For this review, take the finished solid that the model builds, in its own axes (mm). A direction names the side the tool comes from. Round coordinates to 2 decimals unless told otherwise and drop trailing zeros. Write each loop counter-clockwise with the first axis right and the second up, starting at its lowest first coordinate (ties: lowest second). Pieces come first, ordered by that corner, then holes. Notation, with made-up numbers: (49.25, -5) -> (97.25, -5) arc R19 cw to (97.25, 11) -> close; hole circle Ø3 at (67.25, 37). An arc over 180 degrees is marked (long way). Answer as CSV lines item,"result". Start each with the question number.
Item 1: Take a section at D-D on z = -15. Give the boundary of the cut face in (x, y).
Item 2: Take a section at C-C on y = 20.5. Give the boundary of the cut face in (x, z), then the cut area to 3 significant figures.
Item 3: Machinability: for faces 4 (the flat face through (-12, 87, -36.799)), 5 (the flat face through (-10, 11.43, -28)), 6 (the flat face through (-12, 87, -17.749)), which of the approach directions +Z, -Z, +X, -X, +Y, -Y give a long, thin tool a straight path to every point of the face, cutting with its end or side? Answer none if there is none.
Item 4: Take a section at B-B on z = -23. Give the boundary of the cut face in (x, y), then the cut area to 3 significant figures.
Item 5: For pin 1 Ø8 at (y, z) = (43.5, -40.5) entering from +X; pin 2 Ø7 at (x, y) = (-12, 84.5) entering from -Z; pin 3 Ø10 at (x, y) = (-9, 85.5) entering from +Z, all flat-tipped, find the tip position at first contact; note any pin that passes through.
Item 6: Wall thickness on probe 1 along Y at (x, z) = (-16, -25); probe 2 along X at (y, z) = (70, -52); probe 3 along Y at (x, z) = (-16.5, -15): over which ranges is each line inside the solid? List them lowest first. Write a range as from..to.
Item 7: Mouldability with a two-part tool opening along Y and no side actions: class faces 1 (the flat face through (-5.08, 87, -27)), 2 (the flat face through (-11, 83.82, -27)), 3 (the flat face through (-18, 90.17, -28)) as +Y half, -Y half, draft (parallel to the pull), parting line (faces both ways), or undercut.
Item 8: Take a section at A-A on x = -10.5. Give the boundary of the cut face in (y, z).
```python
from build123d import *

# Parameters (mm, degrees)
SKETCH1_W            = 25.4
SKETCH1_H            = 55.88
BOSS_EXTRUDE1_DEPTH  = 11.43
SKETCH3_W            = 6.35
SKETCH3_H            = 55.88
BOSS_EXTRUDE2_DEPTH  = 78.74
SKETCH4_W            = 19.05
SKETCH4_H            = 6.35
BOSS_EXTRUDE3_DEPTH  = 13.97
M3_CLEARANCE_HOLE1_D = 3.6
FILLET1_R            = 2.54


with BuildPart() as part:
    # Sketch1 → Boss-Extrude1 (new body)
    with BuildSketch(Plane(origin=(0, 0, 0), x_dir=(1, 0, 0), z_dir=(0, 1, 0))):
        with Locations((-12.7, 27.94)):
            Rectangle(SKETCH1_W, SKETCH1_H)
    extrude(amount=BOSS_EXTRUDE1_DEPTH)

    # Sketch3 → Boss-Extrude2 (add)
    with BuildSketch(Plane(origin=(0, 11.43, 0), x_dir=(1, 0, 0), z_dir=(0, 1, 0))):
        with Locations((-22.225, 27.94)):
            Rectangle(SKETCH3_W, SKETCH3_H)
    extrude(amount=BOSS_EXTRUDE2_DEPTH)

    # Sketch4 → Boss-Extrude3 (add)
    with BuildSketch(Plane(origin=(-19.05, 0, 0), x_dir=(0, 0, -1), z_dir=(1, 0, 0))):
        with Locations((27.274464597, 86.995)):
            Rectangle(SKETCH4_W, SKETCH4_H)
    extrude(amount=BOSS_EXTRUDE3_DEPTH)

    # M3 Clearance Hole1 (through all)
    with Locations(Plane(origin=(-19.05, 0, 0), x_dir=(0, 0, -1), z_dir=(1, 0, 0))):
        with Locations((4.7625, 48.667276481), (51.1175, 48.667276481)):
            Hole(M3_CLEARANCE_HOLE1_D / 2)

    # Fillet1
    fillet1_edges = [part.edges().sort_by_distance(p)[0] for p in [
        (-19.05, 83.82, -27.274464597),
    ]]
    fillet(fillet1_edges, radius=FILLET1_R)


solid = part.part
```
Output values:
1,outline,"(-25.4, 0) -> (0, 0) -> (0, 11.43) -> (-19.05, 11.43) -> (-19.05, 90.17) -> (-25.4, 90.17) -> close"
2,outline,"(-25.4, -55.88) -> (-19.05, -55.88) -> (-19.05, 0) -> (-25.4, 0) -> close"
2,area,"355 mm^2"
3,face 4,"-Z, +X, +Y"
3,face 5,"+Z, -Z, +X"
3,face 6,"+Z, +X, +Y"
4,outline,"(-25.4, 0) -> (0, 0) -> (0, 11.43) -> (-19.05, 11.43) -> (-19.05, 81.28) arc R2.54 cw to (-16.51, 83.82) -> (-5.08, 83.82) -> (-5.08, 90.17) -> (-25.4, 90.17) -> close"
4,area,"880 mm^2"
5,pin 1,"stops at x = -19.05"
5,pin 2,"stops at z = -36.8"
5,pin 3,"stops at z = -17.75"
6,probe 1,"y = 0..11.43, 83.82..90.17"
6,probe 2,"x = -25.4..-19.05"
6,probe 3,"y = 0..11.43"
7,face 1,"draft"
7,face 2,"undercut"
7,face 3,"+Y half"
8,outline,"(0, -55.88) -> (11.43, -55.88) -> (11.43, 0) -> (0, 0) -> close; (83.82, -36.8) -> (90.17, -36.8) -> (90.17, -17.75) -> (83.82, -17.75) -> close"
